Autodesk Inventor part; units mm, degrees
ref_plane "Plano de trabajo1" through (75, 0, 0) normal (1, 0, 0) x (0, 0, -1)
ref_plane "Plano de trabajo3" through (75, 0, 0) normal (1, 0, 0) x (0, 0, -1)
ref_plane "Plano de trabajo5" through (-10, 75, 144.4118) normal (0, -1, 0) x (1, 0, 0)
sketch "Boceto1" plane through (0, 0, 0) normal (0, 0, 1) x (1, 0, 0)
  line L0 (0, 0) -> (150, 0)
  line L1 (150, 0) -> (150, 150)
  line L2 (150, 150) -> (0, 150)
  line L3 (0, 150) -> (0, 0)
  line L4 (5, 145) -> (145, 145)
  line L5 (145, 145) -> (145, 5)
  line L6 (145, 5) -> (5, 5)
  line L7 (5, 5) -> (5, 145)
  dimension "d0" = 150
  dimension "d1" = 150
  dimension "d2" = 5
extrude "Extrusión1" add sketch "Boceto1" along normal blind 150
sketch "Boceto2" plane through (150, 0, 0) normal (1, 0, 0) x (0, 0, -1)
  line L0 (-150, 0) -> (-150, 150)
  line L1 (-150, 75) -> (-190, 75) construction
  line L2 (-190, 75) -> (-150, 150)
  line L3 (0, 0) -> (-150, 0) construction
  line L4 (-150, 0) -> (-190, 75)
  dimension "d5" = 40
extrude "Extrusión2" add sketch "Boceto2" against normal blind 5
ref_plane "Plano de trabajo1" through (75, 0, 0) normal (1, 0, 0) x (0, 0, -1)
mirror "Simetría1" about plane through (75, 0, 0) normal (1, 0, 0) of "Extrusión2"
sketch "Boceto3" plane through (0, 150, 0) normal (0, 1, 0) x (1, 0, 0)
  line L0 (105, -60) -> (45, -60)
  line L1 (45, -60) -> (45, -95)
  line L2 (60, -110) -> (90, -110)
  line L3 (105, -95) -> (105, -60)
  line L4 (150, 0) -> (0, 0)
  line L5 (145, -150) -> (5, -150)
  arc A0 (90, -110) -> (105, -95) centre (90, -95) ccw
  arc A1 (45, -95) -> (60, -110) centre (60, -95) ccw
  point P0 (45, -110)
  point P1 (105, -110)
  point P2 (75, -60)
  point P3 (75, 0)
  dimension "d8" = 60
  dimension "d9" = 50
  dimension "d10" = 40
  dimension "d11" = 15
extrude "Extrusión3" cut sketch "Boceto3" against normal through all
sketch "Boceto4" plane through (150, 0, 0) normal (1, 0, 0) x (0, 0, -1)
  line L0 (-13, 20) -> (-123, 20)
  line L1 (-128, 25) -> (-128, 75)
  line L2 (-123, 80) -> (-13, 80)
  line L3 (-8, 75) -> (-8, 25)
  line L4 (0, 0) -> (0, 150)
  line L5 (0, 0) -> (-150, 0)
  arc A0 (-123, 80) -> (-128, 75) centre (-123, 75) ccw
  arc A1 (-8, 75) -> (-13, 80) centre (-13, 75) ccw
  arc A2 (-13, 20) -> (-8, 25) centre (-13, 25) ccw
  arc A3 (-128, 25) -> (-123, 20) centre (-123, 25) ccw
  point P0 (-128, 80)
  point P1 (-128, 20)
  point P2 (-8, 80)
  dimension "d14" = 120
  dimension "d15" = 60
  dimension "d16" = 8
  dimension "d17" = 20
  dimension "d18" = 5
extrude "Extrusión4" cut sketch "Boceto4" against normal up to surface (5 mm away)
sketch "Boceto5" plane through (0, 0, 0) normal (-1, 0, 0) x (0, 0, 1)
  line L0 (65, 125) -> (115, 125)
  line L1 (120, 120) -> (120, 30)
  line L2 (115, 25) -> (65, 25)
  line L3 (60, 30) -> (60, 120)
  line L4 (0, 150) -> (0, 0)
  arc A0 (120, 120) -> (115, 125) centre (115, 120) ccw
  arc A1 (115, 25) -> (120, 30) centre (115, 30) ccw
  arc A2 (65, 125) -> (60, 120) centre (65, 120) ccw
  arc A3 (60, 30) -> (65, 25) centre (65, 30) ccw
  point P0 (60, 150)
  point P1 (120, 25)
  point P2 (120, 125)
  point P3 (60, 25)
  point P4 (60, 75)
  point P5 (0, 75)
  dimension "d21" = 60
  dimension "d22" = 100
  dimension "d23" = 60
  dimension "d24" = 5
extrude "Extrusión5" cut sketch "Boceto5" against normal blind 10
sketch "Boceto6" plane through (150, 0, 0) normal (1, 0, 0) x (0, 0, -1)
  line L0 (-190, 75) -> (-150, 0)
  line L1 (-150, 150) -> (-190, 75)
  line L2 (-154.4118, 152.3529) -> (-195.6667, 75)
  line L3 (-195.6667, 75) -> (-154.4118, -2.3529)
  line L4 (-154.4118, 152.3529) -> (-144.4118, 152.3529)
  line L5 (-144.4118, 152.3529) -> (-144.4118, 150)
  line L6 (-154.4118, -2.3529) -> (-144.4118, -2.3529)
  line L7 (-144.4118, -2.3529) -> (-144.4118, 0)
  line L8 (0, 0) -> (-150, 0)
  line L9 (0, 150) -> (-150, 150)
  dimension "d27" = 5
  dimension "d28" = 10
extrude "Extrusión6" add sketch "Boceto6" along normal blind 10 and the other way blind 160
fillet "Empalme1" radius 5 3 edges at (75, 152.3529, 154.4118) (75, 75, 195.6667) (75, -2.3529, 154.4118)
sketch "Boceto8" plane through (150, 0, 0) normal (1, 0, 0) x (0, 0, -1)
  arc A0 (-13, 20) -> (-8, 25) centre (-13, 25) ccw
  line L0 (-13, 20) -> (-123, 20)
  arc A1 (-128, 25) -> (-123, 20) centre (-123, 25) ccw
  line L1 (-128, 25) -> (-128, 75)
  arc A2 (-123, 80) -> (-128, 75) centre (-123, 75) ccw
  line L2 (-123, 80) -> (-13, 80)
  arc A3 (-8, 75) -> (-13, 80) centre (-13, 75) ccw
  line L3 (-8, 75) -> (-8, 25)
  line L4 (0, 0) -> (0, 150)
  line L5 (0, 150) -> (-144.4118, 150)
  line L6 (-144.4118, 150) -> (-150, 150)
  line L7 (-150, 150) -> (-190, 75)
  line L8 (-190, 75) -> (-150, 0)
  line L9 (-144.4118, 0) -> (-150, 0)
  line L10 (0, 0) -> (-144.4118, 0)
  point P0 (0, 0)
extrude "Extrusión8" cut sketch "Boceto8" against normal through all contours L0 A1 L1 A2 L2 A3 L3 A0 | L10 L9 L8 L7 L6 L5 L4
sketch "Boceto9" plane through (160, 0, 150) normal (0, 0.4705882, -0.8823529) x (-1, 0, 0)
  circle A0 centre (12.5, 2.5) radius 1.5
  line L0 (0, 0) -> (0, 85)
  line L1 (170, 0) -> (0, 0)
  point P0 (160, -70.5882)
  dimension "d41" = 3
  dimension "d42" = 12.5
  dimension "d43" = 2.5
extrude "Extrusión9" add sketch "Boceto9" along normal blind 5
ref_plane "Plano de trabajo3" through (75, 0, 0) normal (1, 0, 0) x (0, 0, -1)
mirror "Simetría3" about plane through (75, 0, 0) normal (1, 0, 0) of "Extrusión9"
ref_plane "Plano de trabajo5" through (-10, 75, 144.4118) normal (0, -1, 0) x (1, 0, 0)
mirror "Simetría4" about plane through (-10, 75, 144.4118) normal (0, -1, 0) of "Extrusión9", "Simetría3"
sketch "Boceto10" plane through (160, 0, 150) normal (0, 0.4705882, -0.8823529) x (-1, 0, 0)
  circle A0 centre (167.5, 2.5) radius 1.5
  line L0 (170, 0) -> (0, 0)
  line L1 (170, 85) -> (170, 0)
  line L2 (0, 85) -> (170, 85)
  point P0 (160, -70.5882)
  dimension "d46" = 3
  dimension "d47" = 2.5
  dimension "d48" = 2.5
extrude "Extrusión10" add sketch "Boceto10" along normal blind 5
mirror "Simetría5" about plane through (-10, 75, 144.4118) normal (0, -1, 0) of "Extrusión10"
sketch "Boceto11" plane through (2.5, 4.5588, 146.7647) normal (0, 0.4705882, -0.8823529) x (-1, 0, 0)
  circle A0 centre (0, 0) radius 1.5
  point P0 (2.5, -73.0882)
extrude "Extrusión11" cut sketch "Boceto11" against normal blind 5
sketch "Boceto12" plane through (2.5, 145.4412, 146.7647) normal (0, -0.4705882, -0.8823529) x (-1, 0, 0)
  circle A0 centre (0, 0) radius 1.5
  point P0 (2.5, -59.2647)
extrude "Extrusión12" cut sketch "Boceto12" against normal blind 5
properties part number "TechoCasa" material "Plástico ABS"
Geometry: final body of the model. Coordinates: model frame, mm. A direction names the side the tool comes from. Round coordinates to 2 decimals unless told otherwise and drop trailing zeros. Write each loop counter-clockwise with the first axis right and the second up, starting at its lowest first coordinate (ties: lowest second). Pieces come first, ordered by that corner, then holes. Notation, with made-up numbers: M 80.25,-23.75 L 125.25,-23.75 A17 cw 125.25,6.25 Z; hole C 79.25,-28 d10. An arc over 180 degrees is marked long. Write item = value, one per line.
Item 1: Pull-direction query (Z, two-part tool) for faces 3 (the face through (73.81, 114.036, 174.848)), 4 (the face through (-8.886, 3.873, 149.272)), 5 (the face through (-10, 87, 185)); classes: pulls with the +Z half, pulls with the -Z half, needs draft (parallel to the pull), parting line crosses it, or undercut.
Findings:
face_3 = pulls with the +Z half
face_4 = undercut
face_5 = needs draft
Item 2: Access query for faces 1 (the face through (74, 150, 147)), 2 (the face through (74, 75, 195)). Directions: +Z, -Z, +X, -X, +Y, -Y. A direction counts if a zero-diameter tool reaches every point of the face in a straight line with its end or side. Return the directions, or none.
Findings:
face_1 = -Z, +X, -X
face_2 = +Z, +X, -X
Item 3: Section query D-D on y = 99. Return loops of the section in (x, z).
Findings:
outline = M -10,177.2 L 160,177.2 L 160,182.87 L -10,182.87 Z
Item 4: Section query C-C on z = 184.5. Return loops of the section in (x, y).
Findings:
outline = M -10,54.06 L 160,54.06 L 160,64.69 L -10,64.69 Z; M -10,85.31 L 160,85.31 L 160,95.94 L -10,95.94 Z
Item 5: Section query A-A on x = 36.5. Return loops of the section in (y, z), then the cut area to 3 significant figures.
Findings:
outline = M -2.35,144.41 L 0,144.41 L 0,150 L 75,190 L 150,150 L 150,144.41 L 152.35,144.41 L 152.35,151.41 A5 ccw 149.71,155.82 L 77.35,194.41 A5 ccw 72.65,194.41 L 0.29,155.82 A5 ccw -2.35,151.41 Z
area = 896 mm^2
Item 6: Section query B-B on z = 170.5. Return loops of the section in (x, y), then the cut area to 3 significant figures.
Findings:
outline = M -10,27.81 L 160,27.81 L 160,38.44 L -10,38.44 Z; M -10,111.56 L 160,111.56 L 160,122.19 L -10,122.19 Z
area = 3,610 mm^2
Item 7: Material intervals for line 1 along Y through (x, z) = (104, 171) (3 decimals); line 2 along Y through (x, z) = (5.5, 149); line 3 along Z through (x, y) = (79.5, 74.5), sorted ascending. Write a range as [from, to].
Findings:
line_1 = [28.75, 39.375], [110.625, 121.25]
line_2 = [-2.35, 0], [150, 152.35]
line_3 = [189.73, 194.97]
Item 8: Pin query (flat end, axial travel): P1, Ø8, axis at x = 94.5, y = 111, coming from the -Z side; P2, Ø6, axis at x = 118.5, y = 56, coming from the -Z side; P3, Ø1.5, axis at x = 120.5, y = 37.5, coming from the -Z side. Return the tip coordinate at first contact, or that it passes through.
Findings:
P1 = 168.67
P2 = 178.27
P3 = 169.6
